Source: CAD feature listing. Evaluate the final solid. Frame: model axes, mm. Face numbers are marked on the shaded views. A direction names the side the tool comes from. Give positions to 0.01 mm unless a question says otherwise; leave off trailing zeros. Write each loop counter-clockwise with the first axis right and the second up, starting at its lowest first coordinate (ties: lowest second). Pieces come first, ordered by that corner, then holes.
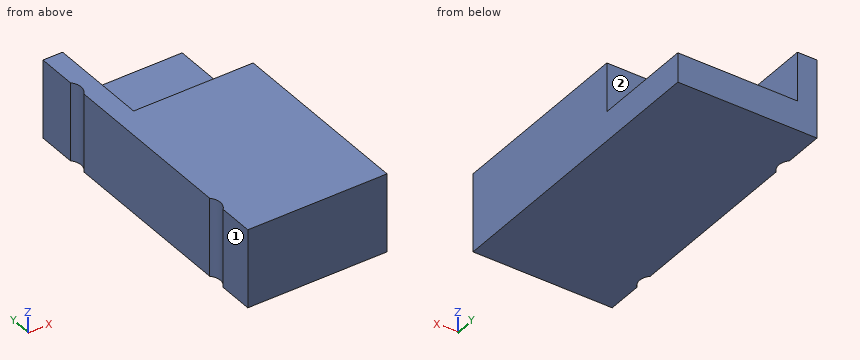
```python
from build123d import *

# Parameters (mm, degrees)
SKETCH1_W           = 18.034
SKETCH1_H           = 38.1
BOSS_EXTRUDE1_DEPTH = 3.81
SKETCH2_W           = 2.54
SKETCH2_H           = 38.1
SKETCH2_H_2         = 24.892
BOSS_EXTRUDE2_DEPTH = 6.35
SKETCH4_W           = 12.954
SKETCH4_H           = 3.17934121
BOSS_EXTRUDE4_DEPTH = 6.35
SKETCH6_R           = 1.778
CUT_EXTRUDE1_DEPTH  = 12.192
SKETCH7_W           = 12.954
SKETCH7_H           = 21.71265879
BOSS_EXTRUDE5_DEPTH = 6.35


with BuildPart() as part:
    # Sketch1 → Boss-Extrude1 (new body)
    with BuildSketch(Plane.XY):
        with Locations((1.952722402, -9.352060056)):
            Rectangle(SKETCH1_W, SKETCH1_H)
    extrude(amount=BOSS_EXTRUDE1_DEPTH)

    # Sketch2 → Boss-Extrude2 (add)
    with BuildSketch(Plane.XY.offset(3.81)):
        with Locations((-5.794277598, -9.352060056)):
            Rectangle(SKETCH2_W, SKETCH2_H)
        with Locations((9.699722402, -15.956060056)):
            Rectangle(SKETCH2_W, SKETCH2_H_2)
    extrude(amount=BOSS_EXTRUDE2_DEPTH)

    # Sketch4 → Boss-Extrude4 (add)
    with BuildSketch(Plane.XY.offset(3.81)):
        with Locations((1.952722402, -5.099730661)):
            Rectangle(SKETCH4_W, SKETCH4_H)
    extrude(amount=BOSS_EXTRUDE4_DEPTH)

    # Sketch6 → Cut-Extrude1 (cut)
    with BuildSketch(Plane.XY):
        with Locations((-8.334277598, 3.347939944)):
            Circle(SKETCH6_R)
        with Locations((-8.334277598, -22.560060056)):
            Circle(SKETCH6_R)
    extrude(amount=CUT_EXTRUDE1_DEPTH, mode=Mode.SUBTRACT)

    # Sketch7 → Boss-Extrude5 (add)
    with BuildSketch(Plane.XY.offset(3.81)):
        with Locations((1.952722402, -17.545730661)):
            Rectangle(SKETCH7_W, SKETCH7_H)
    extrude(amount=BOSS_EXTRUDE5_DEPTH)


solid = part.part
```
1. Access query for the marked faces 1 and 2. Directions: +Z, -Z, +X, -X, +Y, -Y. A direction counts if a zero-diameter tool reaches every point of the face in a straight line with its end or side. Return the directions, or none.
2. Line query: probe 1 along X at (y, z) = (-2, 6.5); probe 2 along Y at (x, z) = (9.75, 6.75); probe 3 along Z at (x, y) = (9.25, 1). Output: solid intervals per line, ascending.
3. Section query C-C (x = 6). Return loops of the section in (y, z).
4. Pin query (flat end, axial travel): P1, Ø3, axis at y = 3, z = 6, coming from the +X side; P2, Ø3, axis at x = 3, z = 6.5, coming from the +Y side; P3, Ø6.5, axis at x = -0.5, y = 0, coming from the +Z side. Return the tip coordinate at first contact, or that it passes through.
5. Section query B-B (z = 5.75). Return loops of the section in (x, y).
6. Section query A-A (y = 1.5). Return loops of the section in (x, z), plus the area to 3 significant figures.
The answers:
1. face 1: +Z, -Z, -X, +Y, -Y
1. face 2: +Z, +X, +Y
2. probe 1: x = -7.06 to -4.52
2. probe 2: y = -28.4 to -3.51
2. probe 3: z = 0 to 3.81
3. outline: (-28.4, 0) - (9.7, 0) - (9.7, 3.81) - (-3.51, 3.81) - (-3.51, 10.16) - (-28.4, 10.16) - close
4. P1: stops at x = -4.52
4. P2: stops at y = -3.51
4. P3: stops at z = 3.81
5. outline: (-7.06, -28.4) - (10.97, -28.4) - (10.97, -3.51) - (-4.52, -3.51) - (-4.52, 9.7) - (-7.06, 9.7) - (-7.06, 4.59) arc R1.78 cw to (-7.06, 2.1) - (-7.06, -21.32) arc R1.78 cw to (-7.06, -23.8) - close
6. outline: (-7.06, 0) - (10.97, 0) - (10.97, 3.81) - (-4.52, 3.81) - (-4.52, 10.16) - (-7.06, 10.16) - close
6. area: 84.8 mm2
